Input: part model. Units: mm. Frame: model coordinates. Round coordinates to 2 decimals unless told otherwise and drop trailing zeros. Loops run counter-clockwise (first coordinate to the right, second up) from the corner with the lowest first, then second, coordinate; pieces in that order, holes last.
1) Section C-C, the plane y = 6.5. Return loops of the section in (x, z).
2) Ray query, line 1 along Y through (x, z) = (-25, 0.4); line 2 along X through (y, z) = (4, 2.95); line 3 along Y through (x, z) = (29, 2.95). Return the intervals inside material, ascending.
3) First-contact query: pin 1 (2 mm diameter, centred on x = 13, z = 3.5, fed in from -Y); pin 2 (1.5 mm diameter, centred on x = 4.5, z = 3, fed in from +Y). Flat tips, straight axial feed; report the tip coordinate or a pass-through.
4) Draft query along Y for faces 1 (the face through (24.1, 39, 2.5)), 2 (the face through (-9.63, 32.31, 2.46)), 3 (the face through (9, 2, 0)), 4 (the face through (19.94, 22.124, 2.465)). Return one class per face: pulls with the +Y half, pulls with the -Y half, needs draft (parallel to the pull), parting line crosses it, or undercut.
5) Section D-D, the plane z = 3.75. State how many separate pieces and enclosed holes the cut face has, and give its area (3 significant figures).
6) Section A-A, the plane y = 21.5. Return loops of the section in (x, z), and give its area (3 significant figures).
7) Section B-B, the plane x = 9. Return loops of the section in (y, z).
from build123d import *

# Parameters (mm, degrees)
ESQUISSE1_R        = 45
ESQUISSE1_R_2      = 13
ESQUISSE1_R_3      = 6
BOSS_EXTRU_1_DEPTH = 5


with BuildPart() as part:
    # Esquisse1 → Boss.-Extru.1 (new body)
    with BuildSketch(Plane.XY):
        with Locations((-0.047735681, 1.026587535)):
            Circle(ESQUISSE1_R)
        with Locations((-0.047735681, 23.526587535)):
            Circle(ESQUISSE1_R_2, mode=Mode.SUBTRACT)
        with Locations((23.526587535, 0.047735681)):
            Circle(ESQUISSE1_R_2, mode=Mode.SUBTRACT)
        with Locations((0.047735681, -23.526587535)):
            Circle(ESQUISSE1_R_2, mode=Mode.SUBTRACT)
        with Locations((-23.526587535, -0.047735681)):
            Circle(ESQUISSE1_R_2, mode=Mode.SUBTRACT)
        with Locations((24.70100166, 25.775324877)):
            Circle(ESQUISSE1_R_3, mode=Mode.SUBTRACT)
        with Locations((25.775324877, -24.70100166)):
            Circle(ESQUISSE1_R_3, mode=Mode.SUBTRACT)
        with Locations((-24.70100166, -25.775324877)):
            Circle(ESQUISSE1_R_3, mode=Mode.SUBTRACT)
        with Locations((-25.775324877, 24.70100166)):
            Circle(ESQUISSE1_R_3, mode=Mode.SUBTRACT)
        with BuildLine():
            Line((-1.565957185, -1.206124597), (1.563345795, -1.140072677))
            ThreePointArc((1.563345795, -1.140072677), (-0.104713375, 3.725986273), (-1.565957185, -1.206124597))
        make_face(mode=Mode.SUBTRACT)
    extrude(amount=BOSS_EXTRU_1_DEPTH)


solid = part.part
Final values:
1. outline: (-44.71, 0) - (-34.76, 0) - (-34.76, 5) - (-44.71, 5) - close; (-12.3, 0) - (12.24, 0) - (12.24, 5) - (-12.3, 5) - close; (34.81, 0) - (44.62, 0) - (44.62, 5) - (34.81, 5) - close
2. line 1: y = -36.42 to -31.77, -19.78 to -12.96, 12.87 to 18.75, 30.65 to 38.48
2. line 2: x = -44.95 to -35.88, -11.17 to 11.14, 35.91 to 44.85
2. line 3: y = -33.34 to -29.76, -19.64 to -11.74, 11.84 to 21.59, 29.96 to 35.4
3. pin 1: stops at y = -42.33
3. pin 2: stops at y = 45.87
4. face 1: parting line crosses it
4. face 2: undercut
4. face 3: needs draft
4. face 4: undercut
5. separate pieces: 1
5. enclosed holes: 9
5. area: 3,760 mm2
6. outline: (-40.12, 0) - (-30.85, 0) - (-30.85, 5) - (-40.12, 5) - close; (-20.7, 0) - (-12.89, 0) - (-12.89, 5) - (-20.7, 5) - close; (12.79, 0) - (20.49, 0) - (20.49, 5) - (12.79, 5) - close; (28.91, 0) - (40.03, 0) - (40.03, 5) - (28.91, 5) - close
6. area: 179 mm2
7. outline: (-43.05, 0) - (-32.95, 0) - (-32.95, 5) - (-43.05, 5) - close; (-14.1, 0) - (14.19, 0) - (14.19, 5) - (-14.1, 5) - close; (32.86, 0) - (45.11, 0) - (45.11, 5) - (32.86, 5) - close
